For this review, take the finished solid that the model builds, in its own axes (mm). Face numbers are marked on the shaded views. A direction names the side the tool comes from. Give positions to 0.01 mm unless a question says otherwise; leave off trailing zeros. Order: outer loops, then holes, each group sorted by start corner. A loop starts at its lowest first (then second) coordinate and runs counter-clockwise, first axis right, second up. Notation, with made-up numbers: (9.25, 11.25) - (32.25, 11.25) arc R34 cw to (32.25, 41.25) - close; hole circle Ø3 at (21.5, 0.5). An arc over 180 degrees is marked (long way). Answer as a JSON object with one key per item and string values. Group by question number.
from build123d import *

# Parameters (mm, degrees)
SKETCH_1_W          = 68
SKETCH_1_H          = 125
EXTRUDE_1_DEPTH     = 3
SKETCH_3_W          = 68
SKETCH_3_H          = 125
SKETCH_3_W_2        = 62
SKETCH_3_H_2        = 119
EXTRUDE_1_2_DEPTH   = 50
FILLET_1_R          = 3
SKETCH_4_W          = 2
SKETCH_4_H          = 10
EXTRUDE_2_DEPTH     = 5
SKETCH_5_R          = 1.75
EXTRUDE_3_DEPTH     = 50
SKETCH_6_R          = 1.75
CUT_EXTRUDE_1_DEPTH = 54


with BuildPart() as part:
    # Эскиз1 → Extrude 1 (new body)
    with BuildSketch(Plane(origin=(0, 0, 0), x_dir=(1, 0, 0), z_dir=(0, 1, 0))):
        Rectangle(SKETCH_1_W, SKETCH_1_H)
    extrude(amount=EXTRUDE_1_DEPTH)

    # Эскиз3 → Extrude 1 2 (add)
    with BuildSketch(Plane(origin=(0, 3, 0), x_dir=(1, 0, 0), z_dir=(0, 1, 0))):
        Rectangle(SKETCH_3_W, SKETCH_3_H)
        Rectangle(SKETCH_3_W_2, SKETCH_3_H_2, mode=Mode.SUBTRACT)
    extrude(amount=EXTRUDE_1_2_DEPTH)

    # Скругление1
    fillet_1_edges = [part.edges().sort_by_distance(p)[0] for p in [
        (-34, 26.5, -62.5),
        (34, 26.5, -62.5),
        (34, 26.5, 62.5),
        (-34, 26.5, 62.5),
    ]]
    fillet(fillet_1_edges, radius=FILLET_1_R)

    # Эскиз4 → Бобышка-Вытянуть2 (add)
    with BuildSketch(Plane(origin=(0, 3, 0), x_dir=(1, 0, 0), z_dir=(0, 1, 0))):
        Polygon((15.75, 11), (25.75, 11), (25.75, 1), (27.75, 1), (27.75, 13), (15.75, 13), align=None)
        with Locations((26.75, -54.5)):
            Rectangle(SKETCH_4_W, SKETCH_4_H)
        with Locations((-26.75, -54.5)):
            Rectangle(SKETCH_4_W, SKETCH_4_H)
        Polygon((-27.75, 13), (-15.75, 13), (-15.75, 11), (-25.75, 11), (-25.75, 1), (-27.75, 1), align=None)
    extrude(amount=EXTRUDE_2_DEPTH)

    # Эскиз5 → Бобышка-Вытянуть3 (add)
    with BuildSketch(Plane(origin=(0, 53, 0), x_dir=(1, 0, 0), z_dir=(0, 1, 0))):
        with BuildLine():
            Line((-29.25, 54.25), (-32.75, 54.25))
            Line((-32.75, 54.25), (-32.75, 57.75))
            ThreePointArc((-32.75, 57.75), (-31.724873734, 60.224873734), (-29.25, 61.25))
            Line((-29.25, 61.25), (-25.75, 61.25))
            Line((-25.75, 61.25), (-25.75, 57.75))
            ThreePointArc((-25.75, 57.75), (-26.775126266, 55.275126266), (-29.25, 54.25))
        make_face()
        with Locations((-29.25, 57.75)):
            Circle(SKETCH_5_R, mode=Mode.SUBTRACT)
        with BuildLine():
            Line((25.75, 61.25), (29.25, 61.25))
            ThreePointArc((29.25, 61.25), (31.724873734, 60.224873734), (32.75, 57.75))
            Line((32.75, 57.75), (32.75, 54.25))
            Line((32.75, 54.25), (29.25, 54.25))
            ThreePointArc((29.25, 54.25), (26.775126266, 55.275126266), (25.75, 57.75))
            Line((25.75, 57.75), (25.75, 61.25))
        make_face()
        with Locations((29.25, 57.75)):
            Circle(SKETCH_5_R, mode=Mode.SUBTRACT)
        with BuildLine():
            Line((29.25, -54.25), (32.75, -54.25))
            Line((32.75, -54.25), (32.75, -57.75))
            ThreePointArc((32.75, -57.75), (31.724873734, -60.224873734), (29.25, -61.25))
            Line((29.25, -61.25), (25.75, -61.25))
            Line((25.75, -61.25), (25.75, -57.75))
            ThreePointArc((25.75, -57.75), (26.775126266, -55.275126266), (29.25, -54.25))
        make_face()
        with Locations((29.25, -57.75)):
            Circle(SKETCH_5_R, mode=Mode.SUBTRACT)
        with BuildLine():
            Line((-25.75, -61.25), (-29.25, -61.25))
            ThreePointArc((-29.25, -61.25), (-31.724873734, -60.224873734), (-32.75, -57.75))
            Line((-32.75, -57.75), (-32.75, -54.25))
            Line((-32.75, -54.25), (-29.25, -54.25))
            ThreePointArc((-29.25, -54.25), (-26.775126266, -55.275126266), (-25.75, -57.75))
            Line((-25.75, -57.75), (-25.75, -61.25))
        make_face()
        with Locations((-29.25, -57.75)):
            Circle(SKETCH_5_R, mode=Mode.SUBTRACT)
    extrude(amount=-EXTRUDE_3_DEPTH)

    # Эскиз6 → Вырез-Вытянуть1 (cut, through all)
    with BuildSketch(Plane(origin=(0, 53, 0), x_dir=(1, 0, 0), z_dir=(0, 1, 0))):
        with Locations((-29.25, 57.75)):
            Circle(SKETCH_6_R)
        with Locations((29.25, 57.75)):
            Circle(SKETCH_6_R)
        with Locations((29.25, -57.75)):
            Circle(SKETCH_6_R)
        with Locations((-29.25, -57.75)):
            Circle(SKETCH_6_R)
    extrude(amount=-CUT_EXTRUDE_1_DEPTH, mode=Mode.SUBTRACT)


solid = part.part
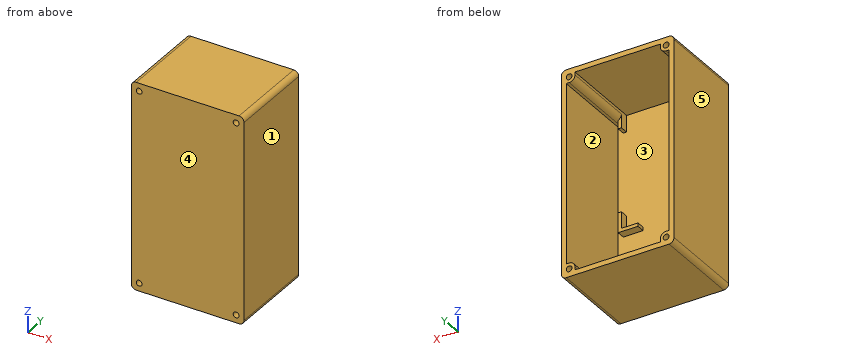
1) Consider section B-B (x = 20). Give the boundary of the cut face in (y, z), plus the area to 3 significant figures.
2) Consider section C-C (z = 8). Give the boundary of the cut face in (x, y).
3) For line 1 (X direction, y = 11, z = 57.75); line 2 (Z direction, x = 29.25, y = 23.5); line 3 (X direction, y = 7.5, z = -5.5), list the stretches that pass through material, from the lowest coordinate up.
4) Consider section A-A (y = 30). Give the boundary of the cut face in (x, z).
5) For the marked faces 1 and 2, list the 3-axis set-ups (+Z, -Z, +X, -X, +Y, -Y) from which the entire face can be reached by the end or side of a thin tool; tool diameter is ignored.
6) For pin 1 (12 mm diameter, centred on x = -10, z = -19, fed in from +Y); pin 2 (2 mm diameter, centred on x = 29.25, z = -57.75, fed in from +Y); pin 3 (1 mm diameter, centred on x = 27, z = 53, fed in from +Y), all flat-tipped, find the tip position at first contact; note any pin that passes through.
7) Consider section D-D (x = 3.5). Give the boundary of the cut face in (y, z).
8) Mouldability with a two-part tool opening along X and no side actions: class the marked faces 3, 4 and 5 as released by +X, released by -X, zero draft, split by the parting line, or undercut.
Result set:
{
 "1": {"outline": "(0, -62.5) - (53, -62.5) - (53, -59.5) - (3, -59.5) - (3, -13) - (8, -13) - (8, -11) - (3, -11) - (3, 59.5) - (53, 59.5) - (53, 62.5) - (0, 62.5) - close", "area": "685 mm2"},
 "2": {"outline": "(-34, 0) - (34, 0) - (34, 53) - (31, 53) - (31, 3) - (-31, 3) - (-31, 53) - (-34, 53) - close"},
 "3": {"line 1": "x = -34 to -31, -27.5 to -25.75, 25.75 to 27.5, 31 to 34", "line 2": "z = -62.5 to -59.5, -56 to -54.25, 54.25 to 56, 59.5 to 62.5", "line 3": "x = -34 to -31, -27.75 to -25.75, 25.75 to 27.75, 31 to 34"},
 "4": {"outline": "(-34, -59.5) arc R3 ccw to (-31, -62.5) - (31, -62.5) arc R3 ccw to (34, -59.5) - (34, 59.5) arc R3 ccw to (31, 62.5) - (-31, 62.5) arc R3 ccw to (-34, 59.5) - close; hole circle Ø3.5 at (-29.25, -57.75); hole (-31, -54.25) - (-29.25, -54.25) arc R3.5 cw to (-25.75, -57.75) - (-25.75, -59.5) - (25.75, -59.5) - (25.75, -57.75) arc R3.5 cw to (29.25, -54.25) - (31, -54.25) - (31, 54.25) - (29.25, 54.25) arc R3.5 cw to (25.75, 57.75) - (25.75, 59.5) - (-25.75, 59.5) - (-25.75, 57.75) arc R3.5 cw to (-29.25, 54.25) - (-31, 54.25) - close; hole circle Ø3.5 at (-29.25, 57.75); hole circle Ø3.5 at (29.25, -57.75); hole circle Ø3.5 at (29.25, 57.75)"},
 "5": {"face 1": "+Z, -Z, +X, +Y, -Y", "face 2": "+Y"},
 "6": {"pin 1": "stops at y = 3", "pin 2": "passes through", "pin 3": "stops at y = 8"},
 "7": {"outline": "(0, -62.5) - (53, -62.5) - (53, -59.5) - (3, -59.5) - (3, 59.5) - (53, 59.5) - (53, 62.5) - (0, 62.5) - close"},
 "8": {"face 3": "undercut", "face 4": "zero draft", "face 5": "released by -X"}
}
